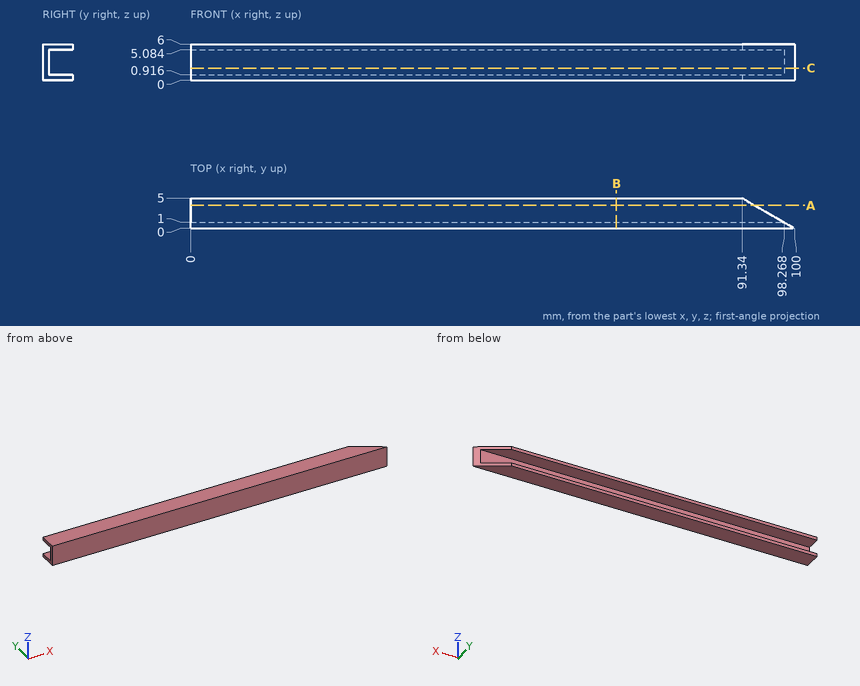
The figure shows three views and two pictorial views of one solid part (mm, origin at its lowest corner). Answer the questions. Coordinates: 2 decimals unless noted, no trailing zeros. Write each loop counter-clockwise with the first axis right and the second up, starting at its lowest first coordinate (ties: lowest second). Pieces come first, ordered by that corner, then holes.
1. The part is cut by section C-C, the plane z = 2. Write down the section's boundary in (x, y).
Results list:
outline: (0, 0) - (100, 0) - (98.27, 1) - (0, 1) - close
2. A flat-ended cylindrical pin translates along its axis: pin 1 (2 mm diameter, centred on x = 59, z = 3, fed in from +Y). Find the tip coordinate at first contact, or state that the pin passes through.
Results list:
pin 1: stops at y = 1
3. Consider line 1 along Z through (x, y) = (70.5, 2.25); line 2 along Y through (x, z) = (86, 4); line 3 along X through (y, z) = (0.6, 4.8). Determine where each line is inside the solid, lowest interval first.
Results list:
line 1: z = 0 to 0.92, 5.08 to 6
line 2: y = 0 to 1
line 3: x = 0 to 98.96
4. The part is cut by section B-B, the plane x = 70.5. Write down the section's boundary in (y, z), and give its area (3 significant figures).
Results list:
outline: (0, 0) - (5, 0) - (5, 0.92) - (1, 0.92) - (1, 5.08) - (5, 5.08) - (5, 6) - (0, 6) - close
area: 13.3 mm2
5. The part is cut by section A-A, the plane y = 3.8. Write down the section's boundary in (x, z), and give its area (3 significant figures).
Results list:
outline: (0, 0) - (93.42, 0) - (93.42, 0.92) - (0, 0.92) - close; (0, 5.08) - (93.42, 5.08) - (93.42, 6) - (0, 6) - close
area: 171 mm2
